Input: part model. Units: mm. Frame: model coordinates. Give positions to 0.01 mm unless a question says otherwise; leave off trailing zeros. Order: outer loops, then holes, each group sorted by start corner. A loop starts at its lowest first (then second) coordinate and runs counter-clockwise, first axis right, second up. Notation, with made-up numbers: (35.25, 18) - (88.25, 18) arc R16 cw to (88.25, 37) - close; hole circle Ø5 at (41, 10.25). An arc over 180 degrees is marked (long way). Use a Markdown table: item, result.
Autodesk Fusion 360 part; units mm, degrees
sketch "Sketch1" plane through (0, 0, 0) normal (0, 0, 1) x (1, 0, 0)
  line L0 (0, 0) -> (336, 0)
  line L1 (336, 0) -> (336, 120)
  line L2 (336, 120) -> (0, 120)
  line L3 (0, 120) -> (0, 0)
  line L4 (10, 110) -> (326, 110)
  line L5 (326, 110) -> (326, 10)
  line L6 (326, 10) -> (10, 10)
  line L7 (10, 10) -> (10, 110)
  line L8 (298, 110) -> (298, 10)
  line L9 (298, 10) -> (326, 10)
  line L10 (326, 10) -> (326, 110)
  line L11 (298.6, 106.03) -> (325.3, 106.03)
  line L12 (325.3, 106.03) -> (325.3, 86.73)
  line L13 (325.3, 86.73) -> (298.6, 86.73)
  line L14 (298.6, 86.73) -> (298.6, 106.03)
  circle A0 centre (6, 114) radius 1
  circle A1 centre (330, 114) radius 1
  circle A2 centre (330, 6) radius 1
  circle A3 centre (6, 6) radius 1
  circle A4 centre (168, 5) radius 1
  circle A5 centre (168, 115) radius 1
  dimension "d1" = 120
  dimension "d2" = 336
  dimension "d3" = 10
  dimension "d4" = 10
  dimension "d5" = 10
  dimension "d6" = 10
  dimension "d7" = 28
  dimension "d8" = 19.3
  dimension "d9" = 0.7
  dimension "d10" = 26.7
  dimension "d11" = 3.97
  dimension "d16" = 2
  dimension "d17" = 6
  dimension "d18" = 6
  dimension "d19" = 2
  dimension "d20" = 6
  dimension "d21" = 6
  dimension "d22" = 2
  dimension "d23" = 6
  dimension "d24" = 6
  dimension "d25" = 2
  dimension "d26" = 6
  dimension "d27" = 6
  dimension "d28" = 2
  dimension "d29" = 168
  dimension "d30" = 2
  dimension "d31" = 168
sketch "Sketch4" plane through (0, 0, 0) normal (0, 0, 1) x (1, 0, 0)
  line L0 (319.15, 77.73) -> (307.75, 77.73)
  line L1 (307.75, 77.73) -> (307.75, 16.73)
  line L2 (307.75, 16.73) -> (319.15, 16.73)
  line L3 (319.15, 16.73) -> (319.15, 77.73)
  line L4 (319.15, 77.73) -> (319.15, 80.98)
  line L5 (319.15, 80.98) -> (323.95, 80.98)
  line L6 (323.95, 80.98) -> (323.95, 69.98)
  line L7 (323.95, 69.98) -> (319.15, 69.98)
  line L8 (319.15, 69.98) -> (319.15, 80.98)
  dimension "d50" = 11.4
  dimension "d51" = 61
  dimension "d52" = 3.25
  dimension "d53" = 4.8
  dimension "d54" = 11
extrude "Extrude3" add sketch "Sketch1" along normal blind 5 contours L0 L1 L2 L3
extrude "Extrude4" add sketch "Sketch1" along normal blind 5 contours L4 L5 L6 L8 L9 L10
extrude "Extrude5" cut sketch "Sketch1" along normal blind 2 contours L4 L5 L6 L8 L9 L10
extrude "Extrude6" cut sketch "Sketch4" along normal blind 5
fillet "Fillet5" radius 5 1 edges at (336, 0, 2.5)
fillet "Fillet6" radius 5 1 edges at (336, 120, 2.5)
fillet "Fillet7" radius 5 1 edges at (0, 120, 2.5)
fillet "Fillet8" radius 5 1 edges at (0, 0, 2.5)
extrude "Extrude1" [suppressed]
extrude "Extrude2" [suppressed]
fillet "Fillet1" [suppressed]
fillet "Fillet2" [suppressed]
fillet "Fillet3" [suppressed]
fillet "Fillet4" [suppressed]
1. Section query A-A (y = 62). Return loops of the section in (x, z).
Response:
| item | result |
|---|---|
| outline | (0, 0) - (10, 0) - (10, 5) - (0, 5) - close; (298, 2) - (307.75, 2) - (307.75, 5) - (298, 5) - close; (319.15, 2) - (326, 2) - (326, 0) - (336, 0) - (336, 5) - (319.15, 5) - close |
2. Section query C-C (z = 0.85). Return loops of the section in (x, y), then the cut area to 3 significant figures.
Response:
| item | result |
|---|---|
| outline | (0, 5) arc R5 ccw to (5, 0) - (331, 0) arc R5 ccw to (336, 5) - (336, 115) arc R5 ccw to (331, 120) - (5, 120) arc R5 ccw to (0, 115) - close; hole circle Ø2 at (6, 6); hole circle Ø2 at (6, 114); hole (10, 10) - (326, 10) - (326, 110) - (10, 110) - close; hole circle Ø2 at (168, 5); hole circle Ø2 at (168, 115); hole circle Ø2 at (330, 6); hole circle Ø2 at (330, 114) |
| area | 8,680 mm^2 |
3. Mould query, pull axis X, two halves, no side actions, for faces 1 (the face through (167, 7, 0)), 2 (the face through (306, 50, 2)). Classes: pulls with the +X half, pulls with the -X half, needs draft (parallel to the pull), parting line crosses it, or undercut.
Response:
| item | result |
|---|---|
| face 1 | needs draft |
| face 2 | undercut |
4. Material intervals for line 1 along X through (y, z) = (34.5, 4.2); line 2 along Y through (x, z) = (6, 3.5); line 3 along X through (y, z) = (88, 4.4), sorted ascending.
Response:
| item | result |
|---|---|
| line 1 | x = 0 to 10, 298 to 307.75, 319.15 to 336 |
| line 2 | y = 0 to 5, 7 to 113, 115 to 120 |
| line 3 | x = 0 to 10, 298 to 298.6, 325.3 to 336 |
5. Section query B-B (x = 26). Return loops of the section in (y, z).
Response:
| item | result |
|---|---|
| outline | (0, 0) - (10, 0) - (10, 5) - (0, 5) - close; (110, 0) - (120, 0) - (120, 5) - (110, 5) - close |
